Work out the finished part from the listing and answer in its coordinate system (mm). A direction names the side the tool comes from. Coordinates: 2 decimals unless noted, no trailing zeros. Order: outer loops, then holes, each group sorted by start corner. A loop starts at its lowest first (then second) coordinate and runs counter-clockwise, first axis right, second up. Notation, with made-up numbers: (-22, 19.5) -> (21, 19.5) arc R23 ccw to (21, 27.5) -> close; hole circle Ø1 at (-18.75, 11). An arc over 180 degrees is marked (long way). Write item = value, one per line. Start each with the question number.
Q1. Which of the six approach directions +Z, -Z, +X, -X, +Y, -Y give full straight-line access (tool end or side, diameter ignored) to faces 4 (the flat face through (-22, 124.92, 28)), 5 (the flat face through (-21, -1156, 29.769)), 6 (the flat face through (-22, -539, 25.387))?
Q2. Straight lines are drawn through the part: L1, parallel to X at y = -908, z = 5; L2, parallel to Z at x = -17.5, y = -1041.5; L3, parallel to Z at x = -22.5, y = -1106. For each, find the intervals that lie inside material, in ascending order. Write a range as from..to.
Q3. The part is cut by section A-A, the plane z = 12.5. Determine the outline of the cut face in (x, y), plus the area to 4 significant figures.
Q4. Flat-ended cylindrical pins translate along their axes: pin 1 (1.5 mm diameter, centred on x = -17, y = -513, fed in from -Z); pin 2 (6 mm diameter, centred on x = -21.59, y = -802.18, fed in from -Z); pin 3 (1.8 mm diameter, centred on x = -30, z = 32.5, fed in from -Y); pin 4 (5 mm diameter, centred on x = -6, y = -573.5, fed in from -Z). Find the tip coordinate at first contact, or state that the pin passes through.
Q5. The part is cut by section B-B, the plane y = -342.5. Determine the outline of the cut face in (x, z).
Q6. For a pull along X with two mould halves and no side action, classify faces 1 (the flat face through (0, -558, 16)), 2 (the flat face through (-18, -1221.28, 26)), 3 (the flat face through (-5.143, -539, 13)) as +X half, -X half, draft (parallel to the pull), parting line (faces both ways), or undercut.
```python
from build123d import *

# Parameters (mm, degrees)
SKETCH1_W                                        = 43.18
SKETCH1_H                                        = 1346.2
BOSS_EXTRUDE1_DEPTH                              = 33.3248
SKETCH9_W                                        = 33.3375
SKETCH9_H                                        = 33.121582444
CUT_EXTRUDE1_DEPTH                               = 1348.304529308
CSK_FOR_10_FLAT_HEAD_MACHINE_SCREW3_D            = 5.1054
CSK_FOR_10_FLAT_HEAD_MACHINE_SCREW3_DEPTH        = 76.2
CSK_FOR_10_FLAT_HEAD_MACHINE_SCREW3_CSINK_D      = 10.2206044
CSK_FOR_10_FLAT_HEAD_MACHINE_SCREW3_CSINK_ANGLE  = 82
CSK_FOR_10_FLAT_HEAD_MACHINE_SCREW3_TIP          = 1.533816902
SKETCH13_W                                       = 3.556
SKETCH13_H                                       = 133.35
CUT_EXTRUDE2_DEPTH                               = 1223.497433688
F_1_4_0_25_DIAMETER_HOLE1_D                      = 6.35
F_1_4_0_25_DIAMETER_HOLE1_DEPTH                  = 101.6
F_1_4_0_25_DIAMETER_HOLE1_TIP                    = 1.907732465
CSK_FOR_1_4_FLAT_HEAD_MACHINE_SCREW1_D           = 6.7564
CSK_FOR_1_4_FLAT_HEAD_MACHINE_SCREW1_CSINK_D     = 13.3194044
CSK_FOR_1_4_FLAT_HEAD_MACHINE_SCREW1_CSINK_ANGLE = 82


with BuildPart() as part:
    # Sketch1 → Boss-Extrude1 (new body)
    with BuildSketch(Plane.XY):
        with Locations((-21.59, -548.180033686)):
            Rectangle(SKETCH1_W, SKETCH1_H)
    extrude(amount=BOSS_EXTRUDE1_DEPTH)

    # Sketch9 → Cut-Extrude1 (cut, through all)
    with BuildSketch(Plane(origin=(0, 124.919966314, 0), x_dir=(1, 0, 0), z_dir=(0, 1, 0))):
        with Locations((-21.81225, -8.826508778)):
            Rectangle(SKETCH9_W, SKETCH9_H)
    extrude(amount=-CUT_EXTRUDE1_DEPTH, mode=Mode.SUBTRACT)

    # CSK for #10 Flat Head Machine Screw3
    with Locations(Plane(origin=(0, 0, 25.3873), x_dir=(-1, 0, 0), z_dir=(0, 0, -1))):
        with Locations((21.59, -1183.180033686), (21.59, -1056.180033686), (21.59, -929.180033686), (21.59, -802.180033686), (21.59, -675.180033686), (21.59, -548.180033686), (21.59, -421.180033686), (21.59, -294.180033686), (21.59, -167.180033686), (21.59, -40.180033686), (21.59, 86.819966314)):
            CounterSinkHole(CSK_FOR_10_FLAT_HEAD_MACHINE_SCREW3_D / 2, CSK_FOR_10_FLAT_HEAD_MACHINE_SCREW3_CSINK_D / 2, depth=CSK_FOR_10_FLAT_HEAD_MACHINE_SCREW3_DEPTH, counter_sink_angle=CSK_FOR_10_FLAT_HEAD_MACHINE_SCREW3_CSINK_ANGLE)
            with Locations((0, 0, -(CSK_FOR_10_FLAT_HEAD_MACHINE_SCREW3_DEPTH + CSK_FOR_10_FLAT_HEAD_MACHINE_SCREW3_TIP / 2))):  # 118° drill point
                Cone(0, CSK_FOR_10_FLAT_HEAD_MACHINE_SCREW3_D / 2, CSK_FOR_10_FLAT_HEAD_MACHINE_SCREW3_TIP, mode=Mode.SUBTRACT)

    # Sketch13 → Cut-Extrude2 (cut, through all)
    with BuildSketch(Plane(origin=(0, 0, 0), x_dir=(0, 0, -1), z_dir=(1, 0, 0))):
        with Locations((-31.5468, -1154.605033686)):
            Rectangle(SKETCH13_W, SKETCH13_H)
    extrude(amount=-CUT_EXTRUDE2_DEPTH, mode=Mode.SUBTRACT)

    # 1/4 (0.25) Diameter Hole1
    with Locations(Plane(origin=(239.606310056, -1806.580108517, 74.980799953), x_dir=(1.0, -1.0349876365418451e-08, -1.6518326251249117e-10), z_dir=(1.651832625124912e-10, 0, 1.0))):
        with Locations((-270.086317003, 693.250072448), (-231.986317003, 693.250072747), (-270.086316654, 648.800072448), (-231.986316654, 648.800072747), (-270.086316305, 604.350072448), (-231.986316305, 604.350072747)):
            Hole(F_1_4_0_25_DIAMETER_HOLE1_D / 2, depth=F_1_4_0_25_DIAMETER_HOLE1_DEPTH)
            with Locations((0, 0, -(F_1_4_0_25_DIAMETER_HOLE1_DEPTH + F_1_4_0_25_DIAMETER_HOLE1_TIP / 2))):  # 118° drill point
                Cone(0, F_1_4_0_25_DIAMETER_HOLE1_D / 2, F_1_4_0_25_DIAMETER_HOLE1_TIP, mode=Mode.SUBTRACT)

    # CSK for 1/4 Flat Head Machine Screw1 (through all)
    with Locations(Plane(origin=(0, 0, 25.3873), x_dir=(-1, 0, 0), z_dir=(0, 0, -1))):
        with Locations((30.47999989, -1157.780033273), (30.480000001, -1202.230033273), (30.479999779, -1113.330033273)):
            CounterSinkHole(CSK_FOR_1_4_FLAT_HEAD_MACHINE_SCREW1_D / 2, CSK_FOR_1_4_FLAT_HEAD_MACHINE_SCREW1_CSINK_D / 2, counter_sink_angle=CSK_FOR_1_4_FLAT_HEAD_MACHINE_SCREW1_CSINK_ANGLE)


solid = part.part
```
Model answer:
q1.face_4 = +Z, -Z, +X, -X, +Y
q1.face_5 = +Z, +X, -X, -Y
q1.face_6 = -Z, +Y, -Y
q2.L1 = -43.18..-38.48, -5.14..0
q2.L2 = 25.39..33.32
q2.L3 = 25.39..29.77
q3.outline = (-43.18, -1221.28) -> (-38.48, -1221.28) -> (-38.48, 124.92) -> (-43.18, 124.92) -> close; (-5.14, -1221.28) -> (0, -1221.28) -> (0, 124.92) -> (-5.14, 124.92) -> close
q3.area = 13,250 mm2
q4.pin_1 = 25.39
q4.pin_2 = 27.81
q4.pin_3 = -1087.93
q4.pin_4 = 0
q5.outline = (-43.18, 0) -> (-38.48, 0) -> (-38.48, 25.39) -> (-5.14, 25.39) -> (-5.14, 0) -> (0, 0) -> (0, 33.32) -> (-43.18, 33.32) -> close
q6.face_1 = +X half
q6.face_2 = draft
q6.face_3 = undercut
